from build123d import *

# Parameters (mm, degrees)
SKETCH_1_R          = 17.35
SKETCH_1_R_2        = 5.6
EXTRUDE_1_DEPTH     = 3.5
SKETCH_3_R          = 23
SKETCH_3_R_2        = 17.35
EXTRUDE_3_DEPTH     = 12.5
SKETCH_4_R          = 5.6
EXTRUDE_4_DEPTH     = 1.1
SKETCH_6_R          = 1
CUT_EXTRUDE_3_DEPTH = 5
SKETCH_8_R          = 1.91
CUT_EXTRUDE_4_DEPTH = 1.9


with BuildPart() as part:
    # 草图1 → 凸台-拉伸1 (new body)
    with BuildSketch(Plane(origin=(0, 0, 0), x_dir=(1, 0, 0), z_dir=(0, 1, 0))):
        with Locations(Location((0, 0, 0), (0, 0, 270))):
            Circle(SKETCH_1_R)
        with Locations(Location((0, 0, 0), (0, 0, 270))):
            Circle(SKETCH_1_R_2, mode=Mode.SUBTRACT)
    extrude(amount=EXTRUDE_1_DEPTH)

    # 草图3 → 凸台-拉伸3 (add)
    with BuildSketch(Plane(origin=(0, 0, 0), x_dir=(1, 0, 0), z_dir=(0, 1, 0))):
        with Locations(Location((0, 0, 0), (0, 0, 270))):
            Circle(SKETCH_3_R)
        with Locations(Location((0, 0, 0), (0, 0, 270))):
            Circle(SKETCH_3_R_2, mode=Mode.SUBTRACT)
    extrude(amount=EXTRUDE_3_DEPTH)

    # 草图4 → 凸台-拉伸4 (add)
    with BuildSketch(Plane(origin=(0, 0, 0), x_dir=(1, 0, 0), z_dir=(0, 1, 0))):
        with Locations(Location((0, 0, 0), (0, 0, 270))):
            Circle(SKETCH_4_R)
    extrude(amount=EXTRUDE_4_DEPTH)

    # 草图6 → 切除-拉伸3 (cut, symmetric)
    with BuildSketch(Plane(origin=(0, 0, 0), x_dir=(1, 0, 0), z_dir=(0, 1, 0))):
        with Locations(Location((8.131727984, 8.131727984, 0), (0, 0, 270))):
            Circle(SKETCH_6_R)
        with Locations(Location((7.424621202, -7.424621202, 0), (0, 0, 270))):
            Circle(SKETCH_6_R)
        with Locations(Location((-8.131727984, -8.131727984, 0), (0, 0, 270))):
            Circle(SKETCH_6_R)
        with Locations(Location((-7.424621202, 7.424621202, 0), (0, 0, 270))):
            Circle(SKETCH_6_R)
    extrude(amount=CUT_EXTRUDE_3_DEPTH, both=True, mode=Mode.SUBTRACT)

    # 草图8 → 切除-拉伸4 (cut)
    with BuildSketch(Plane.XZ):
        with Locations(Location((-8.131727984, 8.131727984, 0), (0, 0, 270))):
            Circle(SKETCH_8_R)
        with Locations(Location((7.424621202, 7.424621202, 0), (0, 0, 270))):
            Circle(SKETCH_8_R)
        with Locations(Location((-7.424621202, -7.424621202, 0), (0, 0, 270))):
            Circle(SKETCH_8_R)
        with Locations(Location((8.131727984, -8.131727984, 0), (0, 0, 270))):
            Circle(SKETCH_8_R)
    extrude(amount=-CUT_EXTRUDE_4_DEPTH, mode=Mode.SUBTRACT)


solid = part.part
Build history of the part. All positions in model axes, mm. A direction names the side the tool comes from. Round coordinates to 2 decimals unless told otherwise and drop trailing zeros. Write each loop counter-clockwise with the first axis right and the second up, starting at its lowest first coordinate (ties: lowest second). Pieces come first, ordered by that corner, then holes. Notation, with made-up numbers: M 57,74.25 L 116,74.25 A27 ccw 116,93.25 Z; hole C 89,17 d2. An arc over 180 degrees is marked long. Answer in a Markdown table with one row per item.
1. Which spindle directions (+Z, -Z, +X, -X, +Y, -Y) get a long thin tool onto all of the face, cutting with end or side? Do faces 1 (the face through (6.6, 1.9, 6.6)), 2 (the face through (7.523, 2.689, -8.925)), 3 (the face through (5.21, 7.94, 16.55)). Say none if no direction does.
Geometry check:
| item | result |
|---|---|
| face 1 | -Y |
| face 2 | +Y, -Y |
| face 3 | +Y |
2. Probe L1, parallel to X at y = 9.25, z = 0.5; L2, parallel to X at y = 1, z = 7.5; L3, parallel to Y at x = -6.5, z = -8.5. List the from-to ranges inside material, lowest first. Write a range as [from, to].
Geometry check:
| item | result |
|---|---|
| L1 | [-22.99, -17.34], [17.34, 22.99] |
| L2 | [-21.74, -9.93], [-6.33, 5.52], [9.33, 21.74] |
| L3 | [1.9, 3.5] |
3. Mould opens along Z. For faces 4 (the face through (19.394, 6.162, 12.365)), 5 (the face through (15.4, 12.5, -8.6)), 6 (the face through (10.025, 0.937, -7.883)) say: +Z half, -Z half, draft (parallel to the pull), parting line (faces both ways), or undercut.
Geometry check:
| item | result |
|---|---|
| face 4 | parting line |
| face 5 | draft |
| face 6 | undercut |
4. Saw through at B-B (x = 0). List the corners of the cut face in (y, z).
Geometry check:
| item | result |
|---|---|
| outline | M 0,-23 L 12.5,-23 L 12.5,-17.35 L 3.5,-17.35 L 3.5,-5.6 L 1.1,-5.6 L 1.1,5.6 L 3.5,5.6 L 3.5,17.35 L 12.5,17.35 L 12.5,23 L 0,23 Z |
5. Saw through at C-C (y = 8.5). List the corners of the cut face in (x, z), and give its area (3 significant figures).
Geometry check:
| item | result |
|---|---|
| outline | C 0,0 d46; hole C 0,0 d34.7 |
| area | 716 mm2 |
6. Saw through at A-A (z = 0). List the corners of the cut face in (x, y).
Geometry check:
| item | result |
|---|---|
| outline | M -23,0 L 23,0 L 23,12.5 L 17.35,12.5 L 17.35,3.5 L 5.6,3.5 L 5.6,1.1 L -5.6,1.1 L -5.6,3.5 L -17.35,3.5 L -17.35,12.5 L -23,12.5 Z |
7. Saw through at D-D (z = 15). List the corners of the cut face in (x, y), and give its area (3 significant figures).
Geometry check:
| item | result |
|---|---|
| outline | M -17.44,0 L 17.44,0 L 17.44,12.5 L 8.72,12.5 L 8.72,3.5 L -8.72,3.5 L -8.72,12.5 L -17.44,12.5 Z |
| area | 279 mm2 |
8. Flat gauge pins, fed straight in: P1, Ø3.5, axis at x = -8.13, z = 8.13, coming from the +Y side; P2, Ø3.5, axis at x = 0.5, z = 2.5, coming from the +Y side; P3, Ø4, axis at x = 6.5, y = 2.5, coming from the +Z side. Where does each tip first touch, or does it go through?
Geometry check:
| item | result |
|---|---|
| P1 | y = 3.5 |
| P2 | y = 1.1 |
| P3 | z = 22.56 |
